Read the model definition and answer for the solid it produces. Units are mm, in the model's axes. A direction names the side the tool comes from. Round coordinates to 2 decimals unless told otherwise and drop trailing zeros. Loops run counter-clockwise (first coordinate to the right, second up) from the corner with the lowest first, then second, coordinate; pieces in that order, holes last. Notation, with made-up numbers: (25.25, -39) - (41.25, -39) arc R11 cw to (41.25, -30) - close; hole circle Ø2 at (-39, 41). An arc over 180 degrees is marked (long way). Use one line per item in the form item = value. Start each with the question number.
```python
from build123d import *

# Parameters (mm, degrees)
SKETCH_W                                = 52.9
SKETCH_H                                = 63.06
PAD_DEPTH                               = 0.6
SKETCH001_W                             = 52.9
SKETCH001_H                             = 63.06
SKETCH001_W_2                           = 51.3
SKETCH001_H_2                           = 61.46
PAD001_DEPTH                            = 5.6
POCKET_DEPTH                            = 165.687809
POCKET_LINEARPATTERN_2_DEPTH            = 165.687809
POCKET_LINEARPATTERN_3_DEPTH            = 165.687809
POCKET_LINEARPATTERN_4_DEPTH            = 165.687809
POCKET_MIRRORED_2_DEPTH                 = 165.687809
POCKET_LINEARPATTERN_2_MIRRORED_2_DEPTH = 165.687809
POCKET_LINEARPATTERN_3_MIRRORED_2_DEPTH = 165.687809
POCKET_LINEARPATTERN_4_MIRRORED_2_DEPTH = 165.687809
SKETCH002_R                             = 2.75
PAD002_DEPTH                            = 3.6
SKETCH003_R                             = 1.025
HOLE_DEPTH                              = 171.287809
PAD003_DEPTH                            = 6.3
PAD003_MIRRORED002_2_DEPTH              = 6.3
SKETCH002_MIRRORED002_2_R               = 2.75
PAD002_MIRRORED002_2_DEPTH              = 3.6
SKETCH003_MIRRORED002_2_R               = 1.025
HOLE_MIRRORED002_2_DEPTH                = 171.287809
SKETCH006_R                             = 1.5
PAD004_DEPTH                            = 3
POCKET001_DEPTH                         = 63.061
PAD005_DEPTH                            = 3


with BuildPart() as part:
    # Sketch → Pad (new body)
    with BuildSketch(Plane.XY):
        Rectangle(SKETCH_W, SKETCH_H)
    extrude(amount=PAD_DEPTH)

    # Sketch001 (on Face6 of Pad) → Pad001 (join)
    with BuildSketch(Plane.XY.offset(0.6)):
        Rectangle(SKETCH001_W, SKETCH001_H)
        Rectangle(SKETCH001_W_2, SKETCH001_H_2, mode=Mode.SUBTRACT)
    extrude(amount=PAD001_DEPTH)

    # Sketch005 (on Face6 of Pad) → Pocket (cut, through all)
    with BuildSketch(Plane.XY.offset(0.6)):
        with BuildLine():
            ThreePointArc((-22, 5.5), (-24, 3.5), (-22, 1.5))
            Line((-22, 1.5), (-4, 1.5))
            ThreePointArc((-4, 1.5), (-2, 3.5), (-4, 5.5))
            Line((-4, 5.5), (-22, 5.5))
        make_face()
    pocket = extrude(amount=-POCKET_DEPTH, mode=Mode.SUBTRACT)

    # Sketch005 LinearPattern 2 → Pocket LinearPattern 2 (cut, through all)
    with BuildSketch(Plane(origin=(0, 7, 0.6), x_dir=(1, 0, 0), z_dir=(0, 0, 1))):
        with BuildLine():
            ThreePointArc((-22, 5.5), (-24, 3.5), (-22, 1.5))
            Line((-22, 1.5), (-4, 1.5))
            ThreePointArc((-4, 1.5), (-2, 3.5), (-4, 5.5))
            Line((-4, 5.5), (-22, 5.5))
        make_face()
    pocket_linearpattern_2 = extrude(amount=-POCKET_LINEARPATTERN_2_DEPTH, mode=Mode.SUBTRACT)

    # Sketch005 LinearPattern 3 → Pocket LinearPattern 3 (cut, through all)
    with BuildSketch(Plane(origin=(0, 14, 0.6), x_dir=(1, 0, 0), z_dir=(0, 0, 1))):
        with BuildLine():
            ThreePointArc((-22, 5.5), (-24, 3.5), (-22, 1.5))
            Line((-22, 1.5), (-4, 1.5))
            ThreePointArc((-4, 1.5), (-2, 3.5), (-4, 5.5))
            Line((-4, 5.5), (-22, 5.5))
        make_face()
    pocket_linearpattern_3 = extrude(amount=-POCKET_LINEARPATTERN_3_DEPTH, mode=Mode.SUBTRACT)

    # Sketch005 LinearPattern 4 → Pocket LinearPattern 4 (cut, through all)
    with BuildSketch(Plane(origin=(0, 21, 0.6), x_dir=(1, 0, 0), z_dir=(0, 0, 1))):
        with BuildLine():
            ThreePointArc((-22, 5.5), (-24, 3.5), (-22, 1.5))
            Line((-22, 1.5), (-4, 1.5))
            ThreePointArc((-4, 1.5), (-2, 3.5), (-4, 5.5))
            Line((-4, 5.5), (-22, 5.5))
        make_face()
    pocket_linearpattern_4 = extrude(amount=-POCKET_LINEARPATTERN_4_DEPTH, mode=Mode.SUBTRACT)

    # Sketch005 Mirrored 2 → Pocket Mirrored 2 (cut, through all)
    with BuildSketch(Plane(origin=(0, 0, 0.6), x_dir=(-1, 0, 0), z_dir=(0, 0, -1))):
        with BuildLine():
            ThreePointArc((-22, 5.5), (-24, 3.5), (-22, 1.5))
            Line((-22, 1.5), (-4, 1.5))
            ThreePointArc((-4, 1.5), (-2, 3.5), (-4, 5.5))
            Line((-4, 5.5), (-22, 5.5))
        make_face()
    pocket_mirrored_2 = extrude(amount=POCKET_MIRRORED_2_DEPTH, mode=Mode.SUBTRACT)

    # Sketch005 LinearPattern 2 Mirrored 2 → Pocket LinearPattern 2 Mirrored 2 (cut, through all)
    with BuildSketch(Plane(origin=(0, 7, 0.6), x_dir=(-1, 0, 0), z_dir=(0, 0, -1))):
        with BuildLine():
            ThreePointArc((-22, 5.5), (-24, 3.5), (-22, 1.5))
            Line((-22, 1.5), (-4, 1.5))
            ThreePointArc((-4, 1.5), (-2, 3.5), (-4, 5.5))
            Line((-4, 5.5), (-22, 5.5))
        make_face()
    pocket_linearpattern_2_mirrored_2 = extrude(amount=POCKET_LINEARPATTERN_2_MIRRORED_2_DEPTH, mode=Mode.SUBTRACT)

    # Sketch005 LinearPattern 3 Mirrored 2 → Pocket LinearPattern 3 Mirrored 2 (cut, through all)
    with BuildSketch(Plane(origin=(0, 14, 0.6), x_dir=(-1, 0, 0), z_dir=(0, 0, -1))):
        with BuildLine():
            ThreePointArc((-22, 5.5), (-24, 3.5), (-22, 1.5))
            Line((-22, 1.5), (-4, 1.5))
            ThreePointArc((-4, 1.5), (-2, 3.5), (-4, 5.5))
            Line((-4, 5.5), (-22, 5.5))
        make_face()
    pocket_linearpattern_3_mirrored_2 = extrude(amount=POCKET_LINEARPATTERN_3_MIRRORED_2_DEPTH, mode=Mode.SUBTRACT)

    # Sketch005 LinearPattern 4 Mirrored 2 → Pocket LinearPattern 4 Mirrored 2 (cut, through all)
    with BuildSketch(Plane(origin=(0, 21, 0.6), x_dir=(-1, 0, 0), z_dir=(0, 0, -1))):
        with BuildLine():
            ThreePointArc((-22, 5.5), (-24, 3.5), (-22, 1.5))
            Line((-22, 1.5), (-4, 1.5))
            ThreePointArc((-4, 1.5), (-2, 3.5), (-4, 5.5))
            Line((-4, 5.5), (-22, 5.5))
        make_face()
    pocket_linearpattern_4_mirrored_2 = extrude(amount=POCKET_LINEARPATTERN_4_MIRRORED_2_DEPTH, mode=Mode.SUBTRACT)

    # Mirrored001: Pocket, Pocket LinearPattern 2, Pocket LinearPattern 3, Pocket LinearPattern 4, Pocket Mirrored 2, Pocket LinearPattern 2 Mirrored 2, Pocket LinearPattern 3 Mirrored 2, Pocket LinearPattern 4 Mirrored 2 across Sketch005 H_Axis
    add(pocket.mirror(Plane(origin=(0, 0, 0.6), x_dir=(0, 0, 1), z_dir=(0, 1, 0))), mode=Mode.SUBTRACT)
    add(pocket_linearpattern_2.mirror(Plane(origin=(0, 0, 0.6), x_dir=(0, 0, 1), z_dir=(0, 1, 0))), mode=Mode.SUBTRACT)
    add(pocket_linearpattern_3.mirror(Plane(origin=(0, 0, 0.6), x_dir=(0, 0, 1), z_dir=(0, 1, 0))), mode=Mode.SUBTRACT)
    add(pocket_linearpattern_4.mirror(Plane(origin=(0, 0, 0.6), x_dir=(0, 0, 1), z_dir=(0, 1, 0))), mode=Mode.SUBTRACT)
    add(pocket_mirrored_2.mirror(Plane(origin=(0, 0, 0.6), x_dir=(0, 0, 1), z_dir=(0, 1, 0))), mode=Mode.SUBTRACT)
    add(pocket_linearpattern_2_mirrored_2.mirror(Plane(origin=(0, 0, 0.6), x_dir=(0, 0, 1), z_dir=(0, 1, 0))), mode=Mode.SUBTRACT)
    add(pocket_linearpattern_3_mirrored_2.mirror(Plane(origin=(0, 0, 0.6), x_dir=(0, 0, 1), z_dir=(0, 1, 0))), mode=Mode.SUBTRACT)
    add(pocket_linearpattern_4_mirrored_2.mirror(Plane(origin=(0, 0, 0.6), x_dir=(0, 0, 1), z_dir=(0, 1, 0))), mode=Mode.SUBTRACT)

    # Sketch002 (on Face4 of Pad001) → Pad002 (join)
    with BuildSketch(Plane(origin=(0, 0, 0), x_dir=(1, 0, 0), z_dir=(0, 0, -1))):
        with Locations((22.606, 27.686)):
            Circle(SKETCH002_R)
    pad002 = extrude(amount=-PAD002_DEPTH)

    # Sketch003 (on Face4 of Pad002) → Hole (cut, through all)
    with BuildSketch(Plane(origin=(0, 0, 0), x_dir=(1, 0, 0), z_dir=(0, 0, -1))):
        with Locations((22.606, 27.686)):
            Circle(SKETCH003_R)
    hole = extrude(amount=-HOLE_DEPTH, mode=Mode.SUBTRACT)

    # Sketch004 (on Face10 of Pad001) → Pad003 (join)
    with BuildSketch(Plane.YZ.offset(26.45)):
        Polygon((31.53, 5.7), (30.73, 5.7), (30.38, 6.05), (30.38, 6.25), (30.73, 6.6), (31.53, 6.6), align=None)
    pad003 = extrude(amount=-PAD003_DEPTH)

    # Sketch004 Mirrored002 2 → Pad003 Mirrored002 2 (add)
    with BuildSketch(Plane(origin=(26.45, 0, 0), x_dir=(0, -1, 0), z_dir=(-1, 0, 0))):
        Polygon((31.53, 5.7), (30.73, 5.7), (30.38, 6.05), (30.38, 6.25), (30.73, 6.6), (31.53, 6.6), align=None)
    pad003_mirrored002_2 = extrude(amount=PAD003_MIRRORED002_2_DEPTH)

    # Sketch002 Mirrored002 2 → Pad002 Mirrored002 2 (add)
    with BuildSketch(Plane.XY):
        with Locations((22.606, 27.686)):
            Circle(SKETCH002_MIRRORED002_2_R)
    pad002_mirrored002_2 = extrude(amount=PAD002_MIRRORED002_2_DEPTH)

    # Sketch003 Mirrored002 2 → Hole Mirrored002 2 (cut, through all)
    with BuildSketch(Plane.XY):
        with Locations((22.606, 27.686)):
            Circle(SKETCH003_MIRRORED002_2_R)
    hole_mirrored002_2 = extrude(amount=HOLE_MIRRORED002_2_DEPTH, mode=Mode.SUBTRACT)

    # Mirrored003: Pad003, Pad002, Hole, Pad003 Mirrored002 2, Pad002 Mirrored002 2, Hole Mirrored002 2 across YZ
    add(pad003.mirror(Plane.YZ))
    add(pad002.mirror(Plane.YZ))
    add(hole.mirror(Plane.YZ), mode=Mode.SUBTRACT)
    add(pad003_mirrored002_2.mirror(Plane.YZ))
    add(pad002_mirrored002_2.mirror(Plane.YZ))
    add(hole_mirrored002_2.mirror(Plane.YZ), mode=Mode.SUBTRACT)

    # Sketch006 (on Face78 of MultiTransform001) → Pad004 (join)
    with BuildSketch(Plane.XY.offset(0.6)):
        Circle(SKETCH006_R)
    extrude(amount=PAD004_DEPTH)

    # Sketch007 (on Face80 of Pad004) → Pocket001 (cut, through all)
    with BuildSketch(Plane.XZ.offset(31.53)):
        Polygon((-19.25, 5.2), (-24.25, 10.2), (24.25, 10.2), (19.25, 5.2), align=None)
    extrude(amount=-POCKET001_DEPTH, mode=Mode.SUBTRACT)

    # Sketch008 (on Face78 of Pocket001) → Pad005 (join)
    with BuildSketch(Plane.XY.offset(0.6)):
        with BuildLine():
            ThreePointArc((25.65, 1.5), (24.15, 0), (25.65, -1.5))
            Line((25.65, 1.5), (25.65, -1.5))
        make_face()
    pad005 = extrude(amount=PAD005_DEPTH)

    # Mirrored004: Pad005 across YZ
    add(pad005.mirror(Plane.YZ))


solid = part.part
```
1) For faces 1 (the cylindrical face through (-24, 3.5, 0.3)), 2 (the flat face through (-25, 0, 3.6)), 3 (the flat face through (0, -31.53, 3)), determine the directions among +Z, -Z, +X, -X, +Y, -Y from which every point of the face is accessible in a straight line to the end or side of a thin tool.
2) Determine the mould class of faces 4 (the cylindrical face through (24, 3.5, 0.3)), 5 (the flat face through (0, 0, 0)) for opening direction X: +X half, -X half, draft (parallel to the pull), parting line (faces both ways), or undercut.
3) A cutting plane is placed at A-A on y = -10.5. Write down the section's boundary in (x, z), plus the area to 3 significant figures.
4) Straight lines are drawn through the part: line 1 (Y direction, x = -17, z = 1); line 2 (X direction, y = 3.5, z = 5.5); line 3 (Z direction, x = 23.5, y = 7.5). For each, find the intervals that lie inside material, in ascending order. Write a range as from..to.
5) Flat-ended cylindrical pins translate along their axes: pin 1 (4.5 mm diameter, centred on x = -22.5, y = 28, fed in from +Z); pin 2 (12 mm diameter, centred on x = 6.5, y = 14, fed in from +Z); pin 3 (6 mm diameter, centred on x = -23.5, y = -26.5, fed in from +Z). Find the tip coordinate at first contact, or state that the pin passes through.
6) A cutting plane is placed at D-D on x = -15. Count the separate pieces of the cut face and the enclosed holes in it, plus the area to 3 significant figures.
7) A cutting plane is placed at C-C on y = 0. Write down the section's boundary in (x, z).
8) A cutting plane is placed at B-B on x = 0. Write down the section's boundary in (y, z).
Checks:
q1.face_1 = +Z, -Z
q1.face_2 = +Z
q1.face_3 = +Z, -Z, +X, -X, -Y
q2.face_4 = undercut
q2.face_5 = draft
q3.outline = (-26.45, 0) - (-24, 0) - (-24, 0.6) - (-25.65, 0.6) - (-25.65, 6.2) - (-26.45, 6.2) - close; (-2, 0) - (2, 0) - (2, 0.6) - (-2, 0.6) - close; (24, 0) - (26.45, 0) - (26.45, 6.2) - (25.65, 6.2) - (25.65, 0.6) - (24, 0.6) - close
q3.area = 14.3 mm²
q4.line_1 = -31.53..-30.73, 30.73..31.53
q4.line_2 = -26.45..-25.65, 25.65..26.45
q4.line_3 = 0..0.6
q5.pin_1 = 3.6
q5.pin_2 = 0.6
q5.pin_3 = 6.2
q6.separate_pieces = 9
q6.enclosed_holes = 0
q6.area = 26.0 mm²
q7.outline = (-26.45, 0) - (26.45, 0) - (26.45, 6.2) - (25.65, 6.2) - (25.65, 3.6) - (24.15, 3.6) - (24.15, 0.6) - (1.5, 0.6) - (1.5, 3.6) - (-1.5, 3.6) - (-1.5, 0.6) - (-24.15, 0.6) - (-24.15, 3.6) - (-25.65, 3.6) - (-25.65, 6.2) - (-26.45, 6.2) - close
q8.outline = (-31.53, 0) - (31.53, 0) - (31.53, 5.2) - (30.73, 5.2) - (30.73, 0.6) - (1.5, 0.6) - (1.5, 3.6) - (-1.5, 3.6) - (-1.5, 0.6) - (-30.73, 0.6) - (-30.73, 5.2) - (-31.53, 5.2) - close
